Build history of the part. All positions in model axes, mm. A direction names the side the tool comes from. Coordinates: 2 decimals unless noted, no trailing zeros. Order: outer loops, then holes, each group sorted by start corner. A loop starts at its lowest first (then second) coordinate and runs counter-clockwise, first axis right, second up. Notation, with made-up numbers: (-24.5, 48.25) - (-9.5, 48.25) arc R19 ccw to (-9.5, 85.25) - close; hole circle Ø6 at (47, 71). An arc over 180 degrees is marked (long way). Answer as CSV lines item,"result". Start each with the question number.
from build123d import *

# Parameters (mm, degrees)
SZKIC1_R                    = 2.9
DODANIE_WYCI_GNI_CIE1_DEPTH = 6
SZKIC2_R                    = 1.6
WYTNIJ_WYCI_GNI_CIE1_DEPTH  = 6
SZKIC3_R                    = 2.9
DODANIE_WYCI_GNI_CIE2_DEPTH = 0.5


with BuildPart() as part:
    # Szkic1 → Dodanie-wyciągnięcie1 (new body)
    with BuildSketch(Plane.XY):
        Circle(SZKIC1_R)
    extrude(amount=DODANIE_WYCI_GNI_CIE1_DEPTH)

    # Szkic2 → Wytnij-wyciągnięcie1 (cut)
    with BuildSketch(Plane.XY.offset(6)):
        Circle(SZKIC2_R)
    extrude(amount=-WYTNIJ_WYCI_GNI_CIE1_DEPTH, mode=Mode.SUBTRACT)

    # Szkic3 → Dodanie-wyciągnięcie2 (add)
    with BuildSketch(Plane.XY.offset(6)):
        Circle(SZKIC3_R)
    extrude(amount=DODANIE_WYCI_GNI_CIE2_DEPTH)


solid = part.part
(1) Drop flat-ended pins along their axis: pin 1 Ø2 at (y, z) = (-1.5, 5.5) entering from -X; pin 2 Ø2 at (y, z) = (1.5, 4.5) entering from +X. Give the stop position or say it passes through.
(2) Pull direction X, two halves, no side cores. Call faces 1 (the cylindrical face through (-1.27, -0.97, 3.04)), 2 (the cylindrical face through (-2.9, 0.1, 3.2)), 3 (the flat face through (0, 0, 6.5)): +X half, -X half, draft (parallel to the pull), parting line (faces both ways), or undercut.
(3) Band-saw the part on D-D on z = 1.75. List the corners of the cut face in (x, y).
(4) Probe L1, parallel to Y at x = 0, z = 2.3; L2, parallel to Y at x = -1.35, z = 1.25; L3, parallel to Z at x = -1.1, y = 0.6. List the from-to ranges inside material, lowest first. Write a range as [from, to].
(5) Band-saw the part on A-A on x = 0. List the corners of the cut face in (y, z).
(6) Which spindle directions (+Z, -Z, +X, -X, +Y, -Y) get a long thin tool onto all of the face, cutting with end or side? Do faces 4 (the flat face through (1.25, -1.25, 0)), 5 (the flat face through (0, 0, 6)). Say none if no direction does.
(7) Band-saw the part on C-C on z = 6.25. List the corners of the cut face in (x, y).
Filled in:
1,pin 1,"stops at x = -2.86"
1,pin 2,"stops at x = 2.86"
2,face 1,"undercut"
2,face 2,"parting line"
2,face 3,"draft"
3,outline,"circle Ø5.8 at (0, 0); hole circle Ø3.2 at (0, 0)"
4,L1,"y = [-2.9, -1.6], [1.6, 2.9]"
4,L2,"y = [-2.57, -0.86], [0.86, 2.57]"
4,L3,"z = [6, 6.5]"
5,outline,"(-2.9, 0) - (-1.6, 0) - (-1.6, 6) - (1.6, 6) - (1.6, 0) - (2.9, 0) - (2.9, 6.5) - (-2.9, 6.5) - close"
6,face 4,"-Z, +X, -X, +Y, -Y"
6,face 5,"-Z"
7,outline,"circle Ø5.8 at (0, 0)"
